```python
from build123d import *

# Parameters (mm, degrees)
SKETCH1_W           = 36.1
SKETCH1_H           = 75.1
SKETCH1_W_2         = 20.1
SKETCH1_H_2         = 40.6
BOSS_EXTRUDE1_DEPTH = 4
SKETCH3_W           = 36.1
SKETCH3_H           = 4
BOSS_EXTRUDE3_DEPTH = 29
BOSS_EXTRUDE4_DEPTH = 4
BOSS_EXTRUDE5_DEPTH = 4
SKETCH12_R          = 2
CUT_EXTRUDE2_DEPTH  = 4
SKETCH16_R          = 2.1
CUT_EXTRUDE3_DEPTH  = 61.382199364


with BuildPart() as part:
    # Sketch1 → Boss-Extrude1 (new body)
    with BuildSketch(Plane.XY):
        with Locations((-2.05, -7.45)):
            Rectangle(SKETCH1_W, SKETCH1_H)
        with Locations((-2.05, 0.05)):
            Rectangle(SKETCH1_W_2, SKETCH1_H_2, mode=Mode.SUBTRACT)
    extrude(amount=BOSS_EXTRUDE1_DEPTH)

    # Sketch3 → Boss-Extrude3 (add)
    with BuildSketch(Plane.XY.offset(4)):
        with Locations((-2.05, -47)):
            Rectangle(SKETCH3_W, SKETCH3_H)
    extrude(amount=-BOSS_EXTRUDE3_DEPTH)

    # Sketch9 → Boss-Extrude4 (add)
    with BuildSketch(Plane(origin=(16, 0, 0), x_dir=(0, 0, -1), z_dir=(1, 0, 0))):
        Polygon((0, -7.031601619), (12.585734956, -45), (0, -45), align=None)
    extrude(amount=-BOSS_EXTRUDE4_DEPTH)

    # Sketch11 → Boss-Extrude5 (add)
    with BuildSketch(Plane.ZY.offset(20.1)):
        Polygon((-12.5, -45), (0, -7.003289616), (0, -45), align=None)
    extrude(amount=-BOSS_EXTRUDE5_DEPTH)

    # Sketch12 → Cut-Extrude2 (cut)
    with BuildSketch(Plane(origin=(0, -45, 0), x_dir=(1, 0, 0), z_dir=(0, 1, 0))):
        with Locations(Location((2.57967866, 17.122546138, 0), (0, 0, 270))):
            Circle(SKETCH12_R)
        with Locations(Location((-6.551547439, 7.935229344, 0), (0, 0, 270))):
            Circle(SKETCH12_R)
    extrude(amount=-CUT_EXTRUDE2_DEPTH, mode=Mode.SUBTRACT)

    # Sketch16 → Cut-Extrude3 (cut, through all)
    with BuildSketch(Plane.XY.offset(4)):
        with Locations((-6.6, 25.35)):
            Circle(SKETCH16_R)
        with Locations((2.4, 25.35)):
            Circle(SKETCH16_R)
        with Locations((-6.6, -25.25)):
            Circle(SKETCH16_R)
        with Locations((2.4, -25.25)):
            Circle(SKETCH16_R)
    extrude(amount=-CUT_EXTRUDE3_DEPTH, mode=Mode.SUBTRACT)


solid = part.part
```
Design review of the part built by this model. Coordinates are the model's own, in mm. A direction names the side the tool comes from. Give positions to 0.01 mm unless a question says otherwise; leave off trailing zeros. Write each loop counter-clockwise with the first axis right and the second up, starting at its lowest first coordinate (ties: lowest second). Pieces come first, ordered by that corner, then holes. Notation, with made-up numbers: (81.5, 16) - (112.5, 16) arc R20 cw to (112.5, 39) - close; hole circle Ø1 at (23.5, -2). An arc over 180 degrees is marked (long way). Return JSON: item names as keys, results as strings. Group by question number.
(1) We need section A-A, the plane y = 25.35. Give the boundary of the cut face in (x, z).
(2) Mouldability with a two-part tool opening along X and no side actions: class faces 3 (the flat face through (-2, -20.25, 2)), 4 (the flat face through (-2, 30.1, 2)), 5 (the flat face through (-20.1, -21, -3)), 6 (the flat face through (-12.1, 0, 2)) as +X half, -X half, draft (parallel to the pull), parting line (faces both ways), or undercut.
(3) Insertion check: pin 1 (1 mm diameter, centred on x = 12, z = -19, fed in from +Y); pin 2 (5.5 mm diameter, centred on x = -6.6, y = -25.25, fed in from -Z). Each pin has a flat end and moves straight along its axis. Give the tip position at first contact, or say it passes through.
(4) Machinability: for faces 1 (the flat face through (-2, -45, -12)), 2 (the cylindrical face through (-8.148, 26.769, 2.028)), which of the approach directions +Z, -Z, +X, -X, +Y, -Y give a long, thin tool a straight path to every point of the face, cutting with its end or side? Answer none if there is none.
(5) We need section C-C, the plane x = -7.5. Give the boundary of the cut face in (y, z).
(6) We need section D-D, the plane y = 16.5. Give the boundary of the cut face in (x, z), then the cut area to 3 significant figures.
(7) To check wall thickness, follow probe 1 along Y at (x, z) = (2.4, 1.75); probe 2 along Z at (x, y) = (-6, -41.5); probe 3 along Y at (x, z) = (13, -16). State the ranges of each line that lie inside material, in increasing order.
(8) We need section B-B, the plane z = 0.75. Give the boundary of the cut face in (x, y).
Reported:
{
 "1": {"outline": "(-20.1, 0) - (-8.7, 0) - (-8.7, 4) - (-20.1, 4) - close; (-4.5, 0) - (0.3, 0) - (0.3, 4) - (-4.5, 4) - close; (4.5, 0) - (16, 0) - (16, 4) - (4.5, 4) - close"},
 "2": {"face 3": "undercut", "face 4": "draft", "face 5": "-X half", "face 6": "undercut"},
 "3": {"pin 1": "stops at y = -45", "pin 2": "stops at z = 0"},
 "4": {"face 1": "-Z, +Y", "face 2": "+Z, -Z"},
 "5": {"outline": "(-49, -25) - (-45, -25) - (-45, -9.7) - (-49, -9.7) - close; (-49, -6.17) - (-45, -6.17) - (-45, 0) - (-27.15, 0) - (-27.15, 4) - (-49, 4) - close; (-23.35, 0) - (-20.25, 0) - (-20.25, 4) - (-23.35, 4) - close; (20.35, 0) - (23.45, 0) - (23.45, 4) - (20.35, 4) - close; (27.25, 0) - (30.1, 0) - (30.1, 4) - (27.25, 4) - close"},
 "6": {"outline": "(-20.1, 0) - (-12.1, 0) - (-12.1, 4) - (-20.1, 4) - close; (8, 0) - (16, 0) - (16, 4) - (8, 4) - close", "area": "64.0 mm2"},
 "7": {"probe 1": "y = -49 to -27.35, -23.15 to -20.25, 20.35 to 23.25, 27.45 to 30.1", "probe 2": "z = 0 to 4", "probe 3": "y = -49 to -45"},
 "8": {"outline": "(-20.1, -49) - (16, -49) - (16, 30.1) - (-20.1, 30.1) - close; hole (-12.1, -20.25) - (8, -20.25) - (8, 20.35) - (-12.1, 20.35) - close; hole circle Ø4.2 at (-6.6, -25.25); hole circle Ø4.2 at (-6.6, 25.35); hole circle Ø4.2 at (2.4, -25.25); hole circle Ø4.2 at (2.4, 25.35)"}
}
